Input: part model. Units: mm. Frame: model coordinates. A direction names the side the tool comes from. Coordinates: 2 decimals unless noted, no trailing zeros. Loops run counter-clockwise (first coordinate to the right, second up) from the corner with the lowest first, then second, coordinate; pieces in that order, holes last. Notation, with made-up numbers: M 36.25,45 L 61.25,45 A20 cw 61.25,83 Z; hole C 61.5,-18 d3. An arc over 180 degrees is marked long. Use a Markdown table: item, result. Add a question column.
1. Pin query (flat end, axial travel): pin 1 (8 mm diameter, centred on x = 22, y = 13, fed in from +Z); pin 2 (4.5 mm diameter, centred on x = 12.5, y = 9, fed in from -Z); pin 3 (5 mm diameter, centred on x = 22.5, z = 13, fed in from +Y); pin 4 (8 mm diameter, centred on y = 2.5, z = 16, fed in from +X). Return the tip coordinate at first contact, or that it passes through.
2. Section B-B on x = 12.5. Output: boundary loops of the cut face in (y, z), then the cut area to 4 significant figures.
3. Section A-A on z = 11. Output: boundary loops of the cut face in (x, y).
4. Line query: L1, parallel to Y at x = 12.5, z = 1.25; L2, parallel to Z at x = 23, y = 4.5. Output: solid intervals per line, ascending. Write a range as [from, to].
5. Set-up query: faces 4 (the cylindrical face through (6, 1, 11)), 5 (the flat face through (9.5, 9.4, 1.5)), 6 (the flat face through (25, 1, 6)). Return all of +Z, -Z, +X, -X, +Y, -Y with unobstructed straight access to the full face (end or side cutting, diameter ignored); none if empty.
6. Section D-D on x = 6.5. Output: boundary loops of the cut face in (y, z).
7. Section C-C on y = 9. Output: boundary loops of the cut face in (x, z).
8. Draft query along Z for faces 1 (the flat face through (12, 1, 8.5)), 2 (the cylindrical face through (11, 7, 1)), 3 (the flat face through (9.5, 8.6, 0)). Return one class per face: +Z half, -Z half, draft (parallel to the pull), parting line (faces both ways), or undercut.
```python
from build123d import *

# Parameters (mm, degrees)
SKETCH_1_W          = 25
SKETCH_1_H          = 17
SKETCH_1_R          = 2.5
EXTRUDE_1_DEPTH     = 1.5
SKETCH_2_W          = 25
SKETCH_2_H          = 1.5
EXTRUDE_2_DEPTH     = 19.5
CUT_EXTRUDE_1_DEPTH = 19.5


with BuildPart() as part:
    # 스케치1 → 보스-돌출1 (new body)
    with BuildSketch(Plane.XY):
        with Locations((12.5, 8.5)):
            Rectangle(SKETCH_1_W, SKETCH_1_H)
        with Locations((12.5, 9)):
            Circle(SKETCH_1_R, mode=Mode.SUBTRACT)
    extrude(amount=EXTRUDE_1_DEPTH)

    # 스케치2 → 보스-돌출2 (add)
    with BuildSketch(Plane.XY.offset(1.5)):
        with Locations((12.5, 0.75)):
            Rectangle(SKETCH_2_W, SKETCH_2_H)
    extrude(amount=EXTRUDE_2_DEPTH)

    # 스케치3 → 컷-돌출1 (cut)
    with BuildSketch(Plane(origin=(0, 1.5, 0), x_dir=(1, 0, 0), z_dir=(0, 1, 0))):
        with BuildLine():
            Line((8.5, -8.5), (16.5, -8.5))
            ThreePointArc((16.5, -8.5), (19, -11), (16.5, -13.5))
            Line((16.5, -13.5), (8.5, -13.5))
            ThreePointArc((8.5, -13.5), (6, -11), (8.5, -8.5))
        make_face()
    extrude(amount=-CUT_EXTRUDE_1_DEPTH, mode=Mode.SUBTRACT)


solid = part.part
```
Answers below:
| question | item | result |
|---|---|---|
| 1 | pin 1 | stops at z = 1.5 |
| 1 | pin 2 | passes through |
| 1 | pin 3 | stops at y = 1.5 |
| 1 | pin 4 | stops at x = 25 |
| 2 | outline | M 0,0 L 6.5,0 L 6.5,1.5 L 1.5,1.5 L 1.5,8.5 L 0,8.5 Z; M 0,13.5 L 1.5,13.5 L 1.5,21 L 0,21 Z; M 11.5,0 L 17,0 L 17,1.5 L 11.5,1.5 Z |
| 2 | area | 39.75 mm² |
| 3 | outline | M 0,0 L 6,0 L 6,1.5 L 0,1.5 Z; M 19,0 L 25,0 L 25,1.5 L 19,1.5 Z |
| 4 | L1 | y = [0, 6.5], [11.5, 17] |
| 4 | L2 | z = [0, 1.5] |
| 5 | face 4 | +Y, -Y |
| 5 | face 5 | +Z, +X, -X, +Y |
| 5 | face 6 | +Z, -Z, +X, +Y, -Y |
| 6 | outline | M 0,0 L 17,0 L 17,1.5 L 1.5,1.5 L 1.5,9.5 L 0,9.5 Z; M 0,12.5 L 1.5,12.5 L 1.5,21 L 0,21 Z |
| 7 | outline | M 0,0 L 10,0 L 10,1.5 L 0,1.5 Z; M 15,0 L 25,0 L 25,1.5 L 15,1.5 Z |
| 8 | face 1 | undercut |
| 8 | face 2 | draft |
| 8 | face 3 | -Z half |
